Verification items for the finished model (mm, model axes). Face numbers are marked on the shaded views. A direction names the side the tool comes from. Give positions to 0.01 mm unless a question says otherwise; leave off trailing zeros. Order: outer loops, then holes, each group sorted by start corner. A loop starts at its lowest first (then second) coordinate and runs counter-clockwise, first axis right, second up. Notation, with made-up numbers: (78, 11.5) -> (123, 11.5) arc R27 ccw to (123, 45.5) -> close; hole circle Ø11 at (-5, -2). An arc over 180 degrees is marked (long way). Return JSON: item names as keys, results as strings. Group by question number.
(1) Release check for a two-part mould opening along X. For the marked faces 1, 2, 3 and 4 record: pulls with the +X half, pulls with the -X half, needs draft (parallel to the pull), parting line crosses it, or undercut.
(2) Cross-section at A-A on y = 0. Enter the section's corners in (x, z).
(3) Thickness scan on line 1 along Y through (x, z) = (-1.5, 1.6); line 2 along Y through (x, z) = (-9.5, 4.3); line 3 along X through (y, z) = (1.5, 2.2). Record the ranges inside material, lowest first.
(4) Tool access check on the marked faces 5 and 6. Record the directions out of +Z, -Z, +X, -X, +Y, -Y that give a thin tool (end or side, any length) a straight path to the whole face; none if there is none.
(5) Depth check by flat-ended pin: pin 1 Ø2.5 at (x, z) = (3.5, 1.5) entering from +Y; pin 2 Ø1 at (x, z) = (16, 3) entering from -Y; pin 3 Ø1.8 at (x, y) = (-10.25, 10.25) entering from -Z; pin 4 Ø2.5 at (y, z) = (3.5, 1.5) entering from +X. Enter the tip coordinate at first touch or a pass-through.
(6) Cross-section at C-C on x = 12.5. Enter the section's corners in (y, z), then the cut area to 3 significant figures.
(7) Cross-section at B-B on z = 2.85. Enter the section's corners in (x, y).
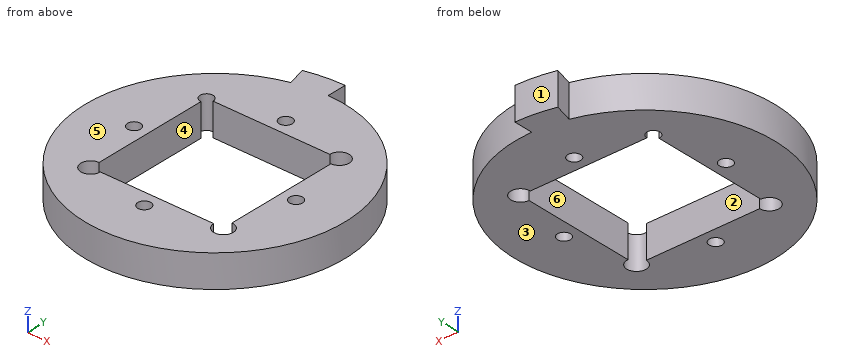
from build123d import *

# Parameters (mm, degrees)
EXTRUDE_1_DEPTH     = 5
SKETCH_2_R          = 1
CUT_EXTRUDE_1_DEPTH = 5


with BuildPart() as part:
    # 草图1 → 凸台-拉伸1 (new body)
    with BuildSketch(Plane.XY):
        with BuildLine():
            ThreePointArc((0, 23), (-3.002102421, 22.803231812), (-5.952838037, 22.216294005))
            Line((-5.952838037, 22.216294005), (-5.176380902, 19.318516526))
            ThreePointArc((-5.176380902, 19.318516526), (2.610523844, -19.828897227), (0, 20))
            Line((0, 20), (0, 23))
        make_face()
        with BuildLine():
            Line((-9.25, 10.25), (8.75, 10.25))
            ThreePointArc((8.75, 10.25), (11.310660172, 11.310660172), (10.25, 8.75))
            Line((10.25, 8.75), (10.25, -8.75))
            ThreePointArc((10.25, -8.75), (11.310660172, -11.310660172), (8.75, -10.25))
            Line((8.75, -10.25), (-8.75, -10.25))
            ThreePointArc((-8.75, -10.25), (-11.310660172, -11.310660172), (-10.25, -8.75))
            Line((-10.25, -8.75), (-10.25, 9.25))
            ThreePointArc((-10.25, 9.25), (-10.957106781, 10.957106781), (-9.25, 10.25))
        make_face(mode=Mode.SUBTRACT)
    extrude(amount=EXTRUDE_1_DEPTH)

    # 草图2 → 切除-拉伸1 (cut)
    with BuildSketch(Plane.XY.offset(5)):
        with Locations((0, 12.5)):
            Circle(SKETCH_2_R)
        with Locations((12.5, 0)):
            Circle(SKETCH_2_R)
        with Locations((0, -12.5)):
            Circle(SKETCH_2_R)
        with Locations((-12.5, 0)):
            Circle(SKETCH_2_R)
    extrude(amount=-CUT_EXTRUDE_1_DEPTH, mode=Mode.SUBTRACT)


solid = part.part
Verdict:
{
 "1": {"face 1": "pulls with the -X half", "face 2": "undercut", "face 3": "needs draft", "face 4": "undercut"},
 "2": {"outline": "(-20, 0) -> (-13.5, 0) -> (-13.5, 5) -> (-20, 5) -> close; (-11.5, 0) -> (-10.25, 0) -> (-10.25, 5) -> (-11.5, 5) -> close; (10.25, 0) -> (11.5, 0) -> (11.5, 5) -> (10.25, 5) -> close; (13.5, 0) -> (20, 0) -> (20, 5) -> (13.5, 5) -> close"},
 "3": {"line 1": "-19.94 to -10.25, 10.25 to 22.95", "line 2": "-17.6 to -11.55, 10.91 to 17.6", "line 3": "-19.94 to -10.25, 10.25 to 19.94"},
 "4": {"face 5": "+Z, +X, -X, +Y, -Y", "face 6": "+Z, -Z"},
 "5": {"pin 1": "y = 19.87", "pin 2": "y = -12.64", "pin 3": "through", "pin 4": "x = 19.87"},
 "6": {"outline": "(-15.61, 0) -> (-1, 0) -> (-1, 5) -> (-15.61, 5) -> close; (1, 0) -> (15.61, 0) -> (15.61, 5) -> (1, 5) -> close", "area": "146 mm²"},
 "7": {"outline": "(-5.95, 22.22) -> (-5.18, 19.32) arc R20 ccw (long way) to (0, 20) -> (0, 23) arc R23 ccw to start; hole circle Ø2 at (-12.5, 0); hole (-10.25, -8.75) arc R1.5 ccw (long way) to (-8.75, -10.25) -> (8.75, -10.25) arc R1.5 ccw (long way) to (10.25, -8.75) -> (10.25, 8.75) arc R1.5 ccw (long way) to (8.75, 10.25) -> (-9.25, 10.25) arc R1 ccw (long way) to (-10.25, 9.25) -> close; hole circle Ø2 at (0, -12.5); hole circle Ø2 at (0, 12.5); hole circle Ø2 at (12.5, 0)"}
}
